Autodesk Inventor part; units mm, degrees
ref_plane "nut_XY" through (0, 0, 0.7493) normal (0, 0, 1) x (1, 0, 0)
ref_plane "nut_YZ" through (0, 0, 0.7493) normal (1, 0, 0) x (0, 1, 0)
ref_plane "nut_ZX" through (0, 0, 0.7493) normal (0, 1, 0) x (0, 0, 1)
sketch "Sketch_1" plane through (0, 0, 0) normal (1, 0, 0) x (0, 1, 0)
  line L0 (0, -0.7493) -> (0, 0.7493)
  line L1 (0, 0.7493) -> (4.0005, 0.7493)
  line L2 (4.0005, 0.7493) -> (4.8006, 0.4581)
  line L3 (4.8006, 0.4581) -> (4.8006, -0.4581)
  line L4 (4.8006, -0.4581) -> (4.0005, -0.7493)
  line L5 (4.0005, -0.7493) -> (0, -0.7493)
  line L6 (0, -0.7493) -> (0, 0.7493)
revolve "Revolution1" add sketch "Sketch_1" angle 360 about axis through (0, 0, -0.7493) along (0, 0, -1)
sketch "Sketch_2" plane through (0, 0, 0) normal (0, 0, 1) x (1, 0, 0)
  line L0 (-8.001, 8.001) -> (-8.001, -8.001)
  line L1 (-8.001, -8.001) -> (8.001, -8.001)
  line L2 (8.001, -8.001) -> (8.001, 8.001)
  line L3 (8.001, 8.001) -> (-8.001, 8.001)
  line L4 (-4.4958, 0) -> (-2.3097, -4.0005)
  line L5 (-2.3097, -4.0005) -> (2.3097, -4.0005)
  line L6 (2.3097, -4.0005) -> (4.4958, 0)
  line L7 (4.4958, 0) -> (2.3097, 4.0005)
  line L8 (2.3097, 4.0005) -> (-2.3097, 4.0005)
  line L9 (-2.3097, 4.0005) -> (-4.4958, 0)
extrude "Extrusion1" cut sketch "Sketch_2" along normal mid plane 2.9972
sketch "Sketch3" plane through (0, 0, -0.7493) normal (0, 0, -1) x (-1, 0, 0)
  point P0 (0, 0)
hole "Drilling 1" at (0, 0, -0.7493) direction (0, 0, 1) diameter 5.3594 depth 1.4986 countersink diameter 6.35 countersink angle 90
ref_plane "nut_XY" through (0, 0, 0.7493) normal (0, 0, 1) x (1, 0, 0)
ref_plane "nut_YZ" through (0, 0, 0.7493) normal (1, 0, 0) x (0, 1, 0)
ref_plane "nut_ZX" through (0, 0, 0.7493) normal (0, 1, 0) x (0, 0, 1)
properties part number "AT513H"
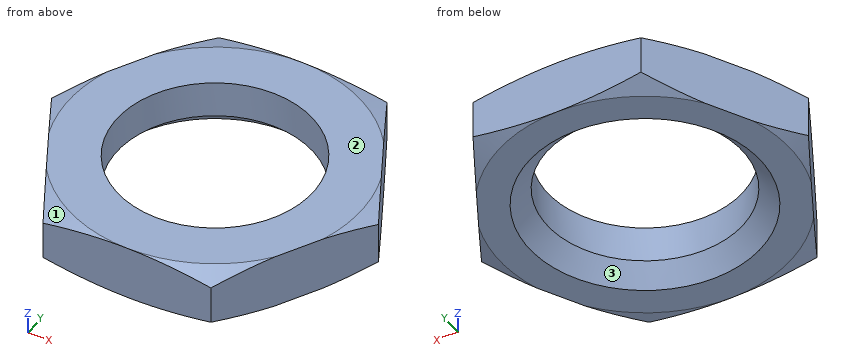
Can you work these out from the model? Positions are in its coordinate system, mm. Face numbers are marked on the shaded views. Coordinates: 2 decimals unless noted, no trailing zeros. Order: outer loops, then holes, each group sorted by start corner. A loop starts at its lowest first (then second) coordinate and runs counter-clockwise, first axis right, second up.
1. Thinking about a two-plate mould opening in Y: for the marked faces 1, 2 and 3, which applies, +Y half, -Y half, draft (parallel to the pull), parting line (faces both ways), or undercut?
2. If we section it at A-A (z = 0.3): Please give me the cut outline in (x, y).
3. I need wall thicknesses on line 1 (Y direction, x = 0, z = 0.45); line 2 (X direction, y = 1.25, z = -0.2); line 3 (Y direction, x = 2, z = -0.2). Which ranges of each line are inside material? Lowest first, please.
Entries:
1. face 1: -Y half
1. face 2: draft
1. face 3: undercut
2. outline: (-4.5, 0) - (-2.31, -4) - (2.31, -4) - (4.5, 0) - (2.31, 4) - (-2.31, 4) - close; hole circle Ø5.36 at (0, 0)
3. line 1: y = -4 to -2.68, 2.68 to 4
3. line 2: x = -3.81 to -2.37, 2.37 to 3.81
3. line 3: y = -4 to -1.78, 1.78 to 4
